Read the model definition and answer for the solid it produces. Units are mm, in the model's axes. A direction names the side the tool comes from. Round coordinates to 2 decimals unless told otherwise and drop trailing zeros. Loops run counter-clockwise (first coordinate to the right, second up) from the corner with the lowest first, then second, coordinate; pieces in that order, holes last. Notation, with made-up numbers: M -23,63 L 32,63 A31 cw 32,88 Z; hole C 56.5,-7 d7. An arc over 180 degrees is marked long. Write each question's results on one line, items separated by ' | '.
Autodesk Fusion 360 part; units mm, degrees
sketch "Boceto1" plane through (0, 0, 0) normal (0, 0, 1) x (1, 0, 0)
  line L0 (0, 0) -> (22, 0)
  line L1 (22, 0) -> (22, 18)
  line L2 (22, 18) -> (0, 18)
  line L3 (0, 18) -> (0, 0)
  dimension "d3" = 22
  dimension "d4" = 18
extrude "Extruir1" add sketch "Boceto1" along normal blind 2
sketch "Boceto2" plane through (0, 0, 0) normal (0, 0, -1) x (1, 0, 0)
  line L0 (0, 0) -> (0, -18)
  line L1 (0, -18) -> (22, -18)
  line L2 (22, -18) -> (22, 0)
  line L3 (22, 0) -> (0, 0)
  line L4 (7.5, 0) -> (9.5, 0)
  line L5 (9.5, 0) -> (9.5, -18)
  line L6 (9.5, -18) -> (7.5, -18)
  line L7 (7.5, -18) -> (7.5, 0)
  line L8 (14.5, 0) -> (12.5, 0)
  line L9 (12.5, 0) -> (12.5, -18)
  line L10 (12.5, -18) -> (14.5, -18)
  line L11 (14.5, -18) -> (14.5, 0)
  dimension "d7" = 2
  dimension "d8" = 2
extrude "Extruir2" add sketch "Boceto2" along normal blind 6 contours L1 L3 L4 L5 L6 L7 | L1 L3 L8 L9 L10 L11
sketch "Boceto3" plane through (14.5, 0, 0) normal (1, 0, 0) x (0, 1, 0)
  line L0 (18, 0) -> (0, 0)
  line L1 (0, 0) -> (0, -6)
  line L2 (0, -6) -> (18, -6)
  line L3 (18, -6) -> (18, 0)
  circle A0 centre (9, -3) radius 1.5
  dimension "d11" = 3
extrude "Extruir3" cut sketch "Boceto3" against normal blind 7 contours A0
sketch "Boceto4" plane through (0, 0, 2) normal (0, 0, 1) x (-1, 0, 0)
  line L0 (0, -18) -> (0, 0)
  line L1 (0, 0) -> (-22, 0)
  line L2 (-22, 0) -> (-22, -18)
  line L3 (-22, -18) -> (0, -18)
  circle A0 centre (-3.4, -4) radius 1.5
  circle A1 centre (-18.5, -4) radius 1.5
  dimension "d14" = 3
  dimension "d15" = 3
extrude "Extruir4" cut sketch "Boceto4" against normal blind 2 contours A0 | A1
1. Determine the mould class of faces 1 (the face through (20, 4, 1)), 2 (the face through (18, 9, 0)), 3 (the face through (3.595, 2.513, 1.014)), 4 (the face through (11, 18, 1)) for opening direction Y: released by +Y, released by -Y, zero draft, split by the parting line, or undercut.
Completed:
face 1: undercut | face 2: zero draft | face 3: undercut | face 4: released by +Y
2. Find the intervals of material crossed by L1, parallel to X at y = 4, z = 0.85; L2, parallel to Y at x = 18.5, z = 1.4; L3, parallel to Z at x = 8.05, y = 9, in increasing order.
Completed:
L1: x = 0 to 1.9, 4.9 to 17, 20 to 22 | L2: y = 0 to 2.5, 5.5 to 18 | L3: z = -6 to -4.5, -1.5 to 2
3. Which of the six approach directions +Z, -Z, +X, -X, +Y, -Y give full straight-line access (tool end or side, diameter ignored) to faces 5 (the face through (14.5, 7, -3)), 6 (the face through (4, 9, 0)), 7 (the face through (9.5, 11, -3))?
Completed:
face 5: -Z, +X, +Y, -Y | face 6: -Z, -X, +Y, -Y | face 7: -Z, +Y, -Y
4. Find section D-D, the plane y = 12.5. Give the vertices of the cut face in (x, z), then the cut area to 3 significant figures.
Completed:
outline: M 0,0 L 7.5,0 L 7.5,-6 L 9.5,-6 L 9.5,0 L 12.5,0 L 12.5,-6 L 14.5,-6 L 14.5,0 L 22,0 L 22,2 L 0,2 Z | area: 68.0 mm2
5. Given P1, Ø2.5, axis at x = 3.4, y = 4, coming from the +Z side; P2, Ø3.5, axis at y = 9, z = -3, coming from the -X side; P3, Ø1.5, axis at x = 11.5, y = 13, coming from the -Z side; P4, Ø3, axis at y = 5, z = -3, coming from the +X side, each flat-ended and moving along its own axis, determine where each tip first touches the part or whether it passes through.
Completed:
P1: passes through | P2: stops at x = 7.5 | P3: stops at z = 0 | P4: stops at x = 14.5
6. Find section A-A, the plane z = -0.75. Give the vertices of the cut face in (x, y).
Completed:
outline: M 7.5,0 L 9.5,0 L 9.5,18 L 7.5,18 Z; M 12.5,0 L 14.5,0 L 14.5,18 L 12.5,18 Z
7. Find section C-C, the plane x = 3.4. Give the vertices of the cut face in (y, z).
Completed:
outline: M 0,0 L 2.5,0 L 2.5,2 L 0,2 Z; M 5.5,0 L 18,0 L 18,2 L 5.5,2 Z
8. Find section B-B, the plane y = 4. Give the vertices of the cut face in (x, z).
Completed:
outline: M 0,0 L 1.9,0 L 1.9,2 L 0,2 Z; M 4.9,0 L 7.5,0 L 7.5,-6 L 9.5,-6 L 9.5,0 L 12.5,0 L 12.5,-6 L 14.5,-6 L 14.5,0 L 17,0 L 17,2 L 4.9,2 Z; M 20,0 L 22,0 L 22,2 L 20,2 Z
